CAD build for the part. Positions are in the model's coordinates, mm. A direction names the side the tool comes from. Round coordinates to 2 decimals unless told otherwise and drop trailing zeros. Write each loop counter-clockwise with the first axis right and the second up, starting at its lowest first coordinate (ties: lowest second). Pieces come first, ordered by that corner, then holes. Notation, with made-up numbers: M 8,-34 L 51,-34 A31 ccw 51,-1 Z; hole C 11.5,33 d4. An arc over 180 degrees is marked long. Write each question's results on one line, items separated by ' | '. Start each with the question number.
```python
from build123d import *

# Parameters (mm, degrees)
SKETCH1_R           = 3.45
SKETCH1_R_2         = 2.1
BOSS_EXTRUDE1_DEPTH = 10
SKETCH2_R           = 1.1
BOSS_EXTRUDE2_DEPTH = 2


with BuildPart() as part:
    # Sketch1 → Boss-Extrude1 (new body)
    with BuildSketch(Plane(origin=(0, 0, 0), x_dir=(1, 0, 0), z_dir=(0, 1, 0))):
        Circle(SKETCH1_R)
        Circle(SKETCH1_R_2, mode=Mode.SUBTRACT)
    extrude(amount=BOSS_EXTRUDE1_DEPTH)

    # Sketch2 → Boss-Extrude2 (add)
    with BuildSketch(Plane(origin=(0, 10, 0), x_dir=(1, 0, 0), z_dir=(0, 1, 0))):
        with BuildLine():
            Line((-3.282257873, 1.215229712), (-0.937787964, 7.547493269))
            ThreePointArc((-0.937787964, 7.547493269), (0, 8.200284779), (0.937787964, 7.547493269))
            Line((0.937787964, 7.547493269), (3.282257873, 1.215229712))
            ThreePointArc((3.282257873, 1.215229712), (3.5, 0), (3.282257873, -1.215229712))
            Line((3.282257873, -1.215229712), (0.937787964, -7.547493269))
            ThreePointArc((0.937787964, -7.547493269), (0, -8.200284779), (-0.937787964, -7.547493269))
            Line((-0.937787964, -7.547493269), (-3.282257873, -1.215229712))
            ThreePointArc((-3.282257873, -1.215229712), (-3.5, 0), (-3.282257873, 1.215229712))
        make_face()
        with Locations((0, -5.6)):
            Circle(SKETCH2_R, mode=Mode.SUBTRACT)
        with Locations((0, 5.6)):
            Circle(SKETCH2_R, mode=Mode.SUBTRACT)
    extrude(amount=BOSS_EXTRUDE2_DEPTH)


solid = part.part
```
1) Saw through at B-B, the plane z = -6. Write the cut outline in (x, y).
2) Wall check: line 1 along X through (y, z) = (6.25, 0); line 2 along Y through (x, z) = (0, 0.5). Give the ranges that are in metal, low to high. Write a range as from..to.
3) Saw through at C-C, the plane y = 1. Write the cut outline in (x, z), plus the area to 3 significant figures.
4) Saw through at D-D, the plane z = 0. Write the cut outline in (x, y), plus the area to 3 significant figures.
5) Saw through at A-A, the plane x = 0. Write the cut outline in (y, z).
6) 3-axis set-ups, long thin cutter, end or side, ignore diameter. For faces 1 (the face through (-3.5, 11, 0)), 2 (the face through (-0.45, 4.93, -3.42)): which of +Z, -Z, +X, -X, +Y, -Y reach the whole face in a straight line?
7) Pull direction Z, two halves, no side cores. Call faces 3 (the face through (3.5, 11, 0)), 4 (the face through (2.003, 4.93, -0.631)), 5 (the face through (2.126, 10.986, 4.337)): pulls with the +Z half, pulls with the -Z half, needs draft (parallel to the pull), parting line crosses it, or undercut.
8) Drop flat-ended pins along their axis: pin 1 Ø2 at (x, z) = (-1.5, 3.5) entering from -Y; pin 2 Ø4 at (y, z) = (3, -6) entering from +X; pin 3 Ø2 at (y, z) = (10, 4) entering from +X; pin 4 Ø3.5 at (x, z) = (0, 0) entering from -Y. Give the stop position or say it passes through.
Filled sheet:
1) outline: M -1.51,10 L -1.02,10 L -1.02,12 L -1.51,12 Z; M 1.02,10 L 1.51,10 L 1.51,12 L 1.02,12 Z
2) line 1: x = -3.45..-2.1, 2.1..3.45 | line 2: y = 10..12
3) outline: C 0,0 d6.9; hole C 0,0 d4.2 | area: 23.5 mm^2
4) outline: M -3.5,10 L -3.45,10 L -3.45,0 L -2.1,0 L -2.1,10 L 2.1,10 L 2.1,0 L 3.45,0 L 3.45,10 L 3.5,10 L 3.5,12 L -3.5,12 Z | area: 41.0 mm^2
5) outline: M 0,-3.45 L 10,-3.45 L 10,-4.5 L 12,-4.5 L 12,4.5 L 10,4.5 L 10,3.45 L 0,3.45 L 0,2.1 L 10,2.1 L 10,-2.1 L 0,-2.1 Z; M 10,-8.2 L 12,-8.2 L 12,-6.7 L 10,-6.7 Z; M 10,6.7 L 12,6.7 L 12,8.2 L 10,8.2 Z
6) face 1: -X, +Y, -Y | face 2: -Y
7) face 3: parting line crosses it | face 4: undercut | face 5: pulls with the +Z half
8) pin 1: stops at y = 0 | pin 2: passes through | pin 3: stops at x = 2.62 | pin 4: stops at y = 10
